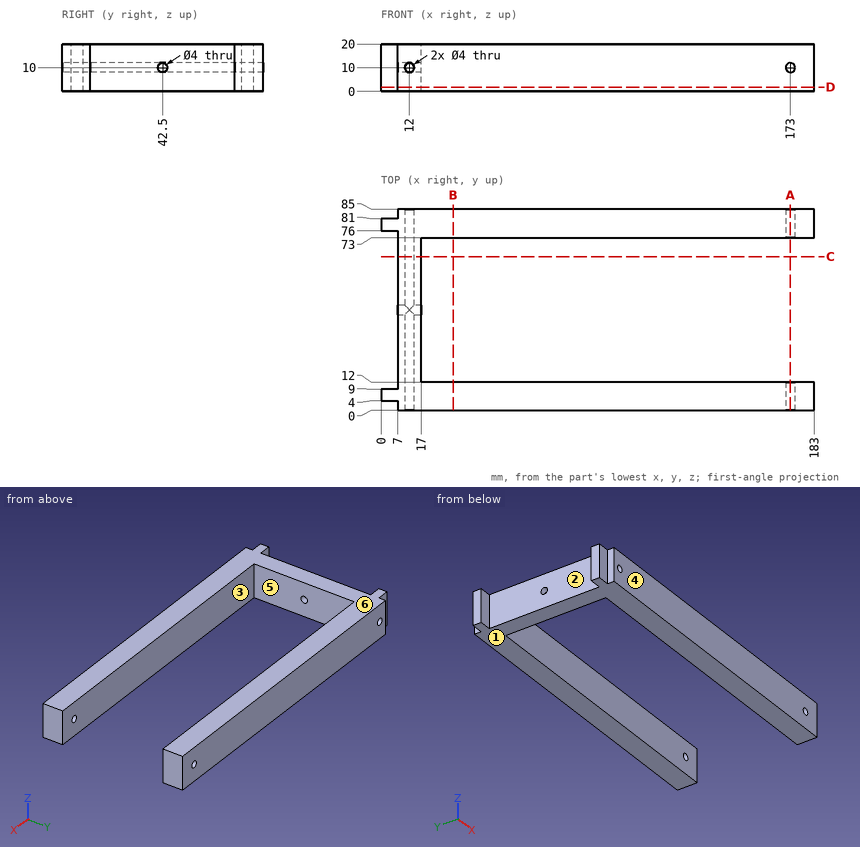
The figure shows three views and two pictorial views of one solid part (mm, origin at its lowest corner). Answer the questions. A direction names the side the tool comes from. Round coordinates to 2 decimals unless told otherwise and drop trailing zeros. Loops run counter-clockwise (first coordinate to the right, second up) from the corner with the lowest first, then second, coordinate; pieces in that order, holes last. Notation, with made-up numbers: M -39.5,-31 L 9.5,-31 A34 ccw 9.5,2 Z; hole C -13,64 d7. An arc over 180 degrees is marked long. Return JSON: item names as keys, results as strings.
Q1. The mould has two halves that part along Y. Classify the marked faces 4, 5 and 6: released by +Y, released by -Y, zero draft, split by the parting line, or undercut.
Results list:
{"face 4": "released by -Y", "face 5": "undercut", "face 6": "zero draft"}
Q2. Find the intervals of material crossed by line 1 along Y through (x, z) = (69.5, 1.5); line 2 along Z through (x, y) = (173, 76); line 3 along X through (y, z) = (17, 10), in increasing order. Write a range as from..to.
Results list:
{"line 1": "y = 0..12, 73..85", "line 2": "z = 0..8, 12..20", "line 3": "x = 7..10, 14..17"}
Q3. Find section D-D, the plane z = 1.75. Determine the outline of the cut face in (x, y), plus the area to 3 significant figures.
Results list:
{"outline": "M 0,4 L 7,4 L 7,0 L 183,0 L 183,12 L 17,12 L 17,73 L 183,73 L 183,85 L 7,85 L 7,81 L 0,81 L 0,76 L 7,76 L 7,9 L 0,9 Z", "area": "4,900 mm2"}
Q4. Which of the six approach directions +Z, -Z, +X, -X, +Y, -Y give full straight-line access (tool end or side, diameter ignored) to the marked faces 1, 2 and 3?
Results list:
{"face 1": "-Z, +X, -X, +Y, -Y", "face 2": "+Z, -Z, -X", "face 3": "+Z, -Z, +X"}
Q5. Find section C-C, the plane y = 65. Determine the outline of the cut face in (x, z), plus the area to 3 significant figures.
Results list:
{"outline": "M 7,0 L 17,0 L 17,20 L 7,20 Z; hole C 12,10 d4", "area": "187 mm2"}
Q6. Each of these flat-tipped pins is pushed along its axis until it touches: pin 1 Ø3 at (x, z) = (12, 10) entering from -Y; pin 2 Ø3 at (y, z) = (83.5, 6.5) entering from -X; pin 3 Ø4.5 at (y, z) = (42.5, 10) entering from +X; pin 4 Ø7.5 at (x, z) = (3, 10) entering from +Y. Where does it stop, or does it pass through?
Results list:
{"pin 1": "passes through", "pin 2": "stops at x = 7", "pin 3": "stops at x = 17", "pin 4": "stops at y = 81"}
Q7. Find section B-B, the plane x = 30.5. Determine the outline of the cut face in (y, z).
Results list:
{"outline": "M 0,0 L 12,0 L 12,20 L 0,20 Z; M 73,0 L 85,0 L 85,20 L 73,20 Z"}
Q8. Find section A-A, the plane x = 173. Determine the outline of the cut face in (y, z), plus the area to 3 significant figures.
Results list:
{"outline": "M 0,0 L 12,0 L 12,8 L 0,8 Z; M 0,12 L 12,12 L 12,20 L 0,20 Z; M 73,0 L 85,0 L 85,8 L 73,8 Z; M 73,12 L 85,12 L 85,20 L 73,20 Z", "area": "384 mm2"}
